from build123d import *

# Parameters (mm, degrees)
ESTRUSIONE_ESTRUSIONE1_DEPTH = 2.5
ESTRUSIONE_ESTRUSIONE2_DEPTH = 15
SCHIZZO2_R                   = 10.25
SCHIZZO2_R_2                 = 2.8
TAGLIO_ESTRUSIONE1_DEPTH     = 15
SCHIZZO3_R                   = 16.1
SCHIZZO3_R_2                 = 14.5
ESTRUSIONE_ESTRUSIONE3_DEPTH = 0.5
SCHIZZO3_3_R                 = 6.3
SCHIZZO3_3_R_2               = 2.25
ESTRUSIONE_ESTRUSIONE4_DEPTH = 3
SCHIZZO3_4_R                 = 5
SCHIZZO3_4_R_2               = 2.8
ESTRUSIONE_ESTRUSIONE5_DEPTH = 5.6
SCHIZZO3_5_R                 = 18.6
SCHIZZO3_5_R_2               = 16.1
ESTRUSIONE_ESTRUSIONE6_DEPTH = 7
SMUSSO1_SIZE                 = 1.5
FORO_PER_VITE_M4_1_D         = 4.5
FORO_PER_VITE_M4_1_DEPTH     = 50
FORO_PER_VITE_M4_1_TIP       = 1.351936393


with BuildPart() as part:
    # Schizzo1 → Estrusione-Estrusione1 (new body)
    with BuildSketch(Plane.XY):
        with BuildLine():
            Line((126, -3.098457484), (126, 38.9))
            Line((126, 38.9), (5.368261151, 38.9))
            ThreePointArc((5.368261151, 38.9), (4.386962529, 38.851736181), (3.415136151, 38.707410603))
            Line((3.415136151, 38.707410603), (-7.887409345, 36.456532663))
            ThreePointArc((-7.887409345, 36.456532663), (-36.456532663, -7.887409345), (7.887409345, -36.456532663))
            Line((7.887409345, -36.456532663), (61.100428827, -16.194450472))
            ThreePointArc((61.100428827, -16.194450472), (93.011370492, -6.976115085), (126, -3.098457484))
        make_face()
        with BuildLine():
            Line((126, 41.4), (5.123487201, 41.4))
            ThreePointArc((5.123487201, 41.4), (4.142188579, 41.351736181), (3.170362201, 41.207410603))
            Line((3.170362201, 41.207410603), (-7.128704932, 39.156373249))
            Line((-7.128704932, 39.156373249), (-8.416056083, 38.9))
            ThreePointArc((-8.416056083, 38.9), (-38.9, -8.416056083), (8.416056083, -38.9))
            Line((8.416056083, -38.9), (61.98889523, -18.531249019))
            ThreePointArc((61.98889523, -18.531249019), (93.463092461, -9.435358059), (126, -5.6))
            Line((126, -5.6), (126, -3.098457484))
            ThreePointArc((126, -3.098457484), (93.011370492, -6.976115085), (61.100428827, -16.194450472))
            Line((61.100428827, -16.194450472), (7.887409345, -36.456532663))
            ThreePointArc((7.887409345, -36.456532663), (-36.456532663, -7.887409345), (-7.887409345, 36.456532663))
            Line((-7.887409345, 36.456532663), (3.415136151, 38.707410603))
            ThreePointArc((3.415136151, 38.707410603), (4.386962529, 38.851736181), (5.368261151, 38.9))
            Line((5.368261151, 38.9), (126, 38.9))
            Line((126, 38.9), (126, 41.4))
        make_face()
    extrude(amount=-ESTRUSIONE_ESTRUSIONE1_DEPTH)

    # Schizzo1<3> → Estrusione-Estrusione2 (add)
    with BuildSketch(Plane.XY):
        with BuildLine():
            Line((126, 41.4), (5.123487201, 41.4))
            ThreePointArc((5.123487201, 41.4), (4.142188579, 41.351736181), (3.170362201, 41.207410603))
            Line((3.170362201, 41.207410603), (-7.128704932, 39.156373249))
            Line((-7.128704932, 39.156373249), (-8.416056083, 38.9))
            ThreePointArc((-8.416056083, 38.9), (-38.9, -8.416056083), (8.416056083, -38.9))
            Line((8.416056083, -38.9), (61.98889523, -18.531249019))
            ThreePointArc((61.98889523, -18.531249019), (93.463092461, -9.435358059), (126, -5.6))
            Line((126, -5.6), (126, -3.098457484))
            ThreePointArc((126, -3.098457484), (93.011370492, -6.976115085), (61.100428827, -16.194450472))
            Line((61.100428827, -16.194450472), (7.887409345, -36.456532663))
            ThreePointArc((7.887409345, -36.456532663), (-36.456532663, -7.887409345), (-7.887409345, 36.456532663))
            Line((-7.887409345, 36.456532663), (3.415136151, 38.707410603))
            ThreePointArc((3.415136151, 38.707410603), (4.386962529, 38.851736181), (5.368261151, 38.9))
            Line((5.368261151, 38.9), (126, 38.9))
            Line((126, 38.9), (126, 41.4))
        make_face()
    extrude(amount=-ESTRUSIONE_ESTRUSIONE2_DEPTH)

    # Schizzo2 → Taglio-Estrusione1 (cut)
    with BuildSketch(Plane.XY):
        Circle(SCHIZZO2_R)
        with Locations((0, -26)):
            Circle(SCHIZZO2_R_2)
        with Locations((0, 26)):
            Circle(SCHIZZO2_R_2)
        with Locations((-26, 0)):
            Circle(SCHIZZO2_R_2)
    extrude(amount=-TAGLIO_ESTRUSIONE1_DEPTH, mode=Mode.SUBTRACT)

    # Schizzo3 → Estrusione-Estrusione3 (add)
    with BuildSketch(Plane(origin=(0, 0, -2.5), x_dir=(-1, 0, 0), z_dir=(0, 0, -1))):
        with Locations(Location((0, 0, 0), (0, 0, 180))):
            Circle(SCHIZZO3_R)
        Circle(SCHIZZO3_R_2, mode=Mode.SUBTRACT)
    extrude(amount=ESTRUSIONE_ESTRUSIONE3_DEPTH)

    # Schizzo3<3> → Estrusione-Estrusione4 (add)
    # profile 1 of 2: a face of its own
    with BuildSketch(Plane(origin=(0, 0, -2.5), x_dir=(-1, 0, 0), z_dir=(0, 0, -1))):
        with Locations(Location((-101, 17.9, 0), (0, 0, 180))):
            Circle(SCHIZZO3_3_R)
        with Locations((-101, 17.9)):
            Circle(SCHIZZO3_3_R_2, mode=Mode.SUBTRACT)
    # profile 2 of 2: a face of its own
    with BuildSketch(Plane(origin=(0, 0, -2.5), x_dir=(-1, 0, 0), z_dir=(0, 0, -1))):
        with Locations(Location((-55, 17.9, 0), (0, 0, 180))):
            Circle(SCHIZZO3_3_R)
        with Locations((-55, 17.9)):
            Circle(SCHIZZO3_3_R_2, mode=Mode.SUBTRACT)
    extrude(amount=ESTRUSIONE_ESTRUSIONE4_DEPTH)

    # Schizzo3<4> → Estrusione-Estrusione5 (add)
    # profile 1 of 4: a face of its own
    with BuildSketch(Plane(origin=(0, 0, -2.5), x_dir=(-1, 0, 0), z_dir=(0, 0, -1))):
        with Locations(Location((0, 26, 0), (0, 0, 180))):
            Circle(SCHIZZO3_4_R)
        with Locations(Location((0, 26, 0), (0, 0, 180))):
            Circle(SCHIZZO3_4_R_2, mode=Mode.SUBTRACT)
    # profile 2 of 4: a face of its own
    with BuildSketch(Plane(origin=(0, 0, -2.5), x_dir=(-1, 0, 0), z_dir=(0, 0, -1))):
        with Locations(Location((26, 0, 0), (0, 0, 180))):
            Circle(SCHIZZO3_4_R)
        with Locations(Location((26, 0, 0), (0, 0, 180))):
            Circle(SCHIZZO3_4_R_2, mode=Mode.SUBTRACT)
    # profile 3 of 4: a face of its own
    with BuildSketch(Plane(origin=(0, 0, -2.5), x_dir=(-1, 0, 0), z_dir=(0, 0, -1))):
        with Locations(Location((-26, 0, 0), (0, 0, 180))):
            Circle(SCHIZZO3_4_R)
        with Locations((-26, 0)):
            Circle(SCHIZZO3_4_R_2, mode=Mode.SUBTRACT)
    # profile 4 of 4: a face of its own
    with BuildSketch(Plane(origin=(0, 0, -2.5), x_dir=(-1, 0, 0), z_dir=(0, 0, -1))):
        with Locations(Location((0, -26, 0), (0, 0, 180))):
            Circle(SCHIZZO3_4_R)
        with Locations(Location((0, -26, 0), (0, 0, 180))):
            Circle(SCHIZZO3_4_R_2, mode=Mode.SUBTRACT)
    extrude(amount=ESTRUSIONE_ESTRUSIONE5_DEPTH)

    # Schizzo3<5> → Estrusione-Estrusione6 (add)
    with BuildSketch(Plane(origin=(0, 0, -2.5), x_dir=(-1, 0, 0), z_dir=(0, 0, -1))):
        with Locations(Location((0, 0, 0), (0, 0, 180))):
            Circle(SCHIZZO3_5_R)
        Circle(SCHIZZO3_5_R_2, mode=Mode.SUBTRACT)
    extrude(amount=ESTRUSIONE_ESTRUSIONE6_DEPTH)

    # Smusso1
    # the kernel refuses this chamfer: 1.5 mm, written as the material it adds along each edge
    with BuildSketch(Plane(origin=(0, 26, -2.5), x_dir=(1, 0, 0), z_dir=(0, 1, 0))) as smusso1_piece_1:
        Polygon((5, SMUSSO1_SIZE), (5 + SMUSSO1_SIZE, 0), (5, 0), align=None)
    revolve(axis=Axis((0, 26, -2.5), (0, 0, -1)))
    with BuildSketch(Plane(origin=(-26, 0, -2.5), x_dir=(1, 0, 0), z_dir=(0, 1, 0))) as smusso1_piece_2:
        Polygon((5, SMUSSO1_SIZE), (5 + SMUSSO1_SIZE, 0), (5, 0), align=None)
    revolve(axis=Axis((-26, 0, -2.5), (0, 0, -1)))
    with BuildSketch(Plane(origin=(26, 0, -2.5), x_dir=(1, 0, 0), z_dir=(0, 1, 0))) as smusso1_piece_3:
        Polygon((5 + SMUSSO1_SIZE, 0), (5, SMUSSO1_SIZE), (5, 0), align=None)
    revolve(axis=Axis((26, 0, -2.5), (0, 0, -1)))
    with BuildSketch(Plane(origin=(0, -26, -2.5), x_dir=(1, 0, 0), z_dir=(0, 1, 0))) as smusso1_piece_4:
        Polygon((5, SMUSSO1_SIZE), (5 + SMUSSO1_SIZE, 0), (5, 0), align=None)
    revolve(axis=Axis((0, -26, -2.5), (0, 0, -1)))
    with BuildSketch(Plane(origin=(0, 0, -2.5), x_dir=(1, 0, 0), z_dir=(0, 1, 0))) as smusso1_piece_5:
        Polygon((18.6, SMUSSO1_SIZE), (18.6 + SMUSSO1_SIZE, 0), (18.6, 0), align=None)
    revolve(axis=Axis((0, 0, -2.5), (0, 0, -1)))
    # the kernel refuses this chamfer: 1.5 mm, written as the material it takes off along each edge
    with BuildSketch(Plane(origin=(55, 17.9, -5.5), x_dir=(1, 0, 0), z_dir=(0, 1, 0))) as smusso1_2_piece_1:
        Polygon((6.3, -SMUSSO1_SIZE), (6.3 - SMUSSO1_SIZE, 0), (6.3, 0), align=None)
    revolve(axis=Axis((55, 17.9, -5.5), (0, 0, -1)), mode=Mode.SUBTRACT)
    with BuildSketch(Plane(origin=(101, 17.9, -5.5), x_dir=(1, 0, 0), z_dir=(0, 1, 0))) as smusso1_2_piece_2:
        Polygon((6.3, -SMUSSO1_SIZE), (6.3 - SMUSSO1_SIZE, 0), (6.3, 0), align=None)
    revolve(axis=Axis((101, 17.9, -5.5), (0, 0, -1)), mode=Mode.SUBTRACT)

    # Foro per Vite M4-1
    with Locations(Plane.XY):
        with Locations((55, 17.9), (101, 17.9)):
            Hole(FORO_PER_VITE_M4_1_D / 2, depth=FORO_PER_VITE_M4_1_DEPTH)
            with Locations((0, 0, -(FORO_PER_VITE_M4_1_DEPTH + FORO_PER_VITE_M4_1_TIP / 2))):  # 118° drill point
                Cone(0, FORO_PER_VITE_M4_1_D / 2, FORO_PER_VITE_M4_1_TIP, mode=Mode.SUBTRACT)


solid = part.part
Model file for the job. Use its own axes, mm. A direction names the side the tool comes from. Give positions to 0.01 mm unless a question says otherwise; leave off trailing zeros. Order: outer loops, then holes, each group sorted by start corner. A loop starts at its lowest first (then second) coordinate and runs counter-clockwise, first axis right, second up. Notation, with made-up numbers: (76, 6) - (80, 6) arc R21 ccw to (80, 17) - close; hole circle Ø10 at (66.25, -13.75). An arc over 180 degrees is marked (long way). One line per item, written item: value.
Item 1: Slice it at D-D (x = 109). List the corners of the cut face in (y, z), then the cut area to 3 significant figures.
Response values:
outline: (-6.93, -15) - (-4.41, -15) - (-4.41, -2.5) - (38.9, -2.5) - (38.9, -15) - (41.4, -15) - (41.4, 0) - (-6.93, 0) - close
area: 184 mm2
Item 2: Slice it at A-A (x = -26). List the corners of the cut face in (y, z).
Response values:
outline: (-30.13, -15) - (-26.74, -15) - (-26.74, -2.5) - (-6.5, -2.5) - (-5, -4) - (-5, -8.1) - (-2.8, -8.1) - (-2.8, 0) - (-30.13, 0) - close; (2.8, -8.1) - (5, -8.1) - (5, -4) - (6.5, -2.5) - (26.74, -2.5) - (26.74, -15) - (30.13, -15) - (30.13, 0) - (2.8, 0) - close
Item 3: Tool access for faces 1 (the flat face through (-2.315, 37.566, -8.662)), 2 (the flat face through (34.866, -26.184, -8.662)), 3 (the cylindrical face through (-28.8, -0.1, -4)): list every direction of +Z, -Z, +X, -X, +Y, -Y with a clear straight run to the whole face (end or side of a thin tool).
Response values:
face 1: -Z, +X
face 2: -Z
face 3: +Z, -Z
Item 4: Pin check, flat tips, straight feed: pin 1 Ø10.5 at (x, y) = (55, 20) entering from -Z; pin 2 Ø5 at (x, y) = (-27, -1) entering from -Z; pin 3 Ø8 at (x, z) = (-5, -8.5) entering from +Y. Stop position of each tip, or through.
Response values:
pin 1: z = -5.5
pin 2: z = -8.1
pin 3: y = 40.38
Item 5: Slice it at C-C (z = -11.5). List the corners of the cut face in (x, y).
Response values:
outline: (-8.42, 38.9) arc R39.8 ccw to (8.42, -38.9) - (61.99, -18.53) arc R200 cw to (126, -5.6) - (126, -3.1) arc R202.5 ccw to (61.1, -16.19) - (7.89, -36.46) arc R37.3 cw to (-7.89, 36.46) - (3.42, 38.71) arc R10 cw to (5.37, 38.9) - (126, 38.9) - (126, 41.4) - (5.12, 41.4) arc R10 ccw to (3.17, 41.21) - close
Item 6: Wall check: line 1 (Y direction, x = -7.5, z = -7.5); line 2 (Y direction, x = 0, z = -1.55); line 3 (Z direction, x = 30.5, y = 27). Give the ranges that are in metal, low to high.
Response values:
line 1: -39.09 to -36.54, -17.02 to -14.25, 14.25 to 17.02, 36.53 to 39.08
line 2: -39.8 to -28.8, -23.2 to -10.25, 10.25 to 23.2, 28.8 to 40.58
line 3: -2.5 to 0
Item 7: Two-plate mould, pull along Y, no slides. Class faces 4 (the cylindrical face through (93.013, -9.527, -7.395)), 5 (the cylindrical face through (28.8, 0.1, -5.3)), 6 (the flat face through (-23.8, 2.2, -8.1)), 7 (the cylindrical face through (-39.076, -7.559, -7.395)): released by +Y, released by -Y, zero draft, split by the parting line, or undercut.
Response values:
face 4: released by -Y
face 5: undercut
face 6: undercut
face 7: split by the parting line
Item 8: Slice it at B-B (y = 26). List the corners of the cut face in (x, z).
Response values:
outline: (-30.13, -15) - (-26.74, -15) - (-26.74, -2.5) - (-6.5, -2.5) - (-5, -4) - (-5, -8.1) - (-2.8, -8.1) - (-2.8, 0) - (-30.13, 0) - close; (2.8, -8.1) - (5, -8.1) - (5, -4) - (6.5, -2.5) - (126, -2.5) - (126, 0) - (2.8, 0) - close
